```python
from build123d import *

# Parameters (mm, degrees)
SKETCH2_W           = 124
SKETCH2_H           = 45
BOSS_EXTRUDE3_DEPTH = 10
SKETCH4_W           = 100
SKETCH4_H           = 45
CUT_EXTRUDE1_DEPTH  = 7
CUT_EXTRUDE2_REACH  = 68.71
SKETCH5_R           = 1.55
SKETCH6_W           = 10.2
SKETCH6_H           = 41.4
CUT_EXTRUDE3_DEPTH  = 7.5
SKETCH7_R           = 1.5
BOSS_EXTRUDE4_DEPTH = 4


with BuildPart() as part:
    # Sketch2 → Boss-Extrude3 (new body)
    with BuildSketch(Plane(origin=(0, 0, 0), x_dir=(1, 0, 0), z_dir=(0, 1, 0))):
        Rectangle(SKETCH2_W, SKETCH2_H)
    extrude(amount=BOSS_EXTRUDE3_DEPTH)

    # Sketch4 → Cut-Extrude1 (cut)
    with BuildSketch(Plane(origin=(0, 10, 0), x_dir=(1, 0, 0), z_dir=(0, 1, 0))):
        Rectangle(SKETCH4_W, SKETCH4_H)
    extrude(amount=-CUT_EXTRUDE1_DEPTH, mode=Mode.SUBTRACT)

    # Sketch5 → Cut-Extrude2 (cut, up to next)
    with BuildSketch(Plane(origin=(0, 10, 0), x_dir=(1, 0, 0), z_dir=(0, 1, 0)), mode=Mode.PRIVATE) as cut_extrude2_sk1:
        with Locations(Location((-57, 12, 0), (0, 0, 270))):
            Circle(SKETCH5_R)
    cut_extrude2_tool1 = extrude(cut_extrude2_sk1.sketch, amount=-CUT_EXTRUDE2_REACH, mode=Mode.PRIVATE) & part.part
    # Sketch5 → Cut-Extrude2 (cut, up to next)
    with BuildSketch(Plane(origin=(0, 10, 0), x_dir=(1, 0, 0), z_dir=(0, 1, 0)), mode=Mode.PRIVATE) as cut_extrude2_sk2:
        with Locations(Location((-57, -12, 0), (0, 0, 270))):
            Circle(SKETCH5_R)
    cut_extrude2_tool2 = extrude(cut_extrude2_sk2.sketch, amount=-CUT_EXTRUDE2_REACH, mode=Mode.PRIVATE) & part.part
    # Sketch5 → Cut-Extrude2 (cut, up to next)
    with BuildSketch(Plane(origin=(0, 10, 0), x_dir=(1, 0, 0), z_dir=(0, 1, 0)), mode=Mode.PRIVATE) as cut_extrude2_sk3:
        with Locations(Location((57, -12, 0), (0, 0, 270))):
            Circle(SKETCH5_R)
    cut_extrude2_tool3 = extrude(cut_extrude2_sk3.sketch, amount=-CUT_EXTRUDE2_REACH, mode=Mode.PRIVATE) & part.part
    # Sketch5 → Cut-Extrude2 (cut, up to next)
    with BuildSketch(Plane(origin=(0, 10, 0), x_dir=(1, 0, 0), z_dir=(0, 1, 0)), mode=Mode.PRIVATE) as cut_extrude2_sk4:
        with Locations(Location((57, 12, 0), (0, 0, 270))):
            Circle(SKETCH5_R)
    cut_extrude2_tool4 = extrude(cut_extrude2_sk4.sketch, amount=-CUT_EXTRUDE2_REACH, mode=Mode.PRIVATE) & part.part
    add(cut_extrude2_tool1.solids().sort_by_distance((-57, 10, -12))[0], mode=Mode.SUBTRACT)
    add(cut_extrude2_tool2.solids().sort_by_distance((-57, 10, 12))[0], mode=Mode.SUBTRACT)
    add(cut_extrude2_tool3.solids().sort_by_distance((57, 10, 12))[0], mode=Mode.SUBTRACT)
    add(cut_extrude2_tool4.solids().sort_by_distance((57, 10, -12))[0], mode=Mode.SUBTRACT)

    # Sketch6 → Cut-Extrude3 (cut)
    with BuildSketch(Plane.XZ):
        with Locations((-56.9, 0)):
            Rectangle(SKETCH6_W, SKETCH6_H)
        with Locations((56.9, 0)):
            Rectangle(SKETCH6_W, SKETCH6_H)
    extrude(amount=-CUT_EXTRUDE3_DEPTH, mode=Mode.SUBTRACT)

    # Sketch7 → Boss-Extrude4 (add)
    # profile 1 of 4: a face of its own
    with BuildSketch(Plane(origin=(0, 3, 0), x_dir=(1, 0, 0), z_dir=(0, 1, 0))):
        with BuildLine():
            Line((-50, -17.5), (-44.5, -17.5))
            Line((-44.5, -17.5), (-44.5, -14.5))
            ThreePointArc((-44.5, -14.5), (-45.232233047, -12.732233047), (-47, -12))
            Line((-47, -12), (-50, -12))
            Line((-50, -12), (-50, -17.5))
        make_face()
        with Locations(Location((-47, -14.5, 0), (0, 0, 270))):
            Circle(SKETCH7_R, mode=Mode.SUBTRACT)
    # profile 2 of 4: a face of its own
    with BuildSketch(Plane(origin=(0, 3, 0), x_dir=(1, 0, 0), z_dir=(0, 1, 0))):
        with BuildLine():
            Line((44.5, -14.5), (44.5, -17.5))
            Line((44.5, -17.5), (50, -17.5))
            Line((50, -17.5), (50, -12))
            Line((50, -12), (47, -12))
            ThreePointArc((47, -12), (45.232233047, -12.732233047), (44.5, -14.5))
        make_face()
        with Locations(Location((47, -14.5, 0), (0, 0, 270))):
            Circle(SKETCH7_R, mode=Mode.SUBTRACT)
    # profile 3 of 4: a face of its own
    with BuildSketch(Plane(origin=(0, 3, 0), x_dir=(1, 0, 0), z_dir=(0, 1, 0))):
        with BuildLine():
            Line((-50, 17.5), (-50, 12))
            Line((-50, 12), (-47, 12))
            ThreePointArc((-47, 12), (-45.232233047, 12.732233047), (-44.5, 14.5))
            Line((-44.5, 14.5), (-44.5, 17.5))
            Line((-44.5, 17.5), (-50, 17.5))
        make_face()
        with Locations(Location((-47, 14.5, 0), (0, 0, 270))):
            Circle(SKETCH7_R, mode=Mode.SUBTRACT)
    # profile 4 of 4: a face of its own
    with BuildSketch(Plane(origin=(0, 3, 0), x_dir=(1, 0, 0), z_dir=(0, 1, 0))):
        with BuildLine():
            Line((47, 12), (50, 12))
            Line((50, 12), (50, 17.5))
            Line((50, 17.5), (44.5, 17.5))
            Line((44.5, 17.5), (44.5, 14.5))
            ThreePointArc((44.5, 14.5), (45.232233047, 12.732233047), (47, 12))
        make_face()
        with Locations(Location((47, 14.5, 0), (0, 0, 270))):
            Circle(SKETCH7_R, mode=Mode.SUBTRACT)
    extrude(amount=BOSS_EXTRUDE4_DEPTH)


solid = part.part
```
Check sheet for the modelled part. Datum: model origin and axes. Units: mm. A direction names the side the tool comes from. Coordinates: 2 decimals unless noted, no trailing zeros. Write each loop counter-clockwise with the first axis right and the second up, starting at its lowest first coordinate (ties: lowest second). Pieces come first, ordered by that corner, then holes. Notation, with made-up numbers: (48, -5) -> (98, -5) arc R14 cw to (98, 1) -> close; hole circle Ø11 at (66.5, 12.25). An arc over 180 degrees is marked (long way). Use a Markdown table: item, result.
1. Tool access check on faces 4 (the flat face through (44.5, 5, -16)), 5 (the cylindrical face through (-48.464, 4.972, -14.825)), 6 (the flat face through (-47, 5, 17.5)). Record the directions out of +Z, -Z, +X, -X, +Y, -Y that give a thin tool (end or side, any length) a straight path to the whole face; none if there is none.
Reported:
| item | result |
|---|---|
| face 4 | +Z, -Z, +Y |
| face 5 | +Y |
| face 6 | +Z, +Y |
2. Sectioned sample at D-D (x = 33.5). Enter the section's corners in (y, z), plus the area to 3 significant figures.
Reported:
| item | result |
|---|---|
| outline | (0, -22.5) -> (3, -22.5) -> (3, 22.5) -> (0, 22.5) -> close |
| area | 135 mm2 |
3. Sectioned sample at C-C (z = 1.5). Enter the section's corners in (x, y), plus the area to 3 significant figures.
Reported:
| item | result |
|---|---|
| outline | (-62, 7.5) -> (-51.8, 7.5) -> (-51.8, 0) -> (51.8, 0) -> (51.8, 7.5) -> (62, 7.5) -> (62, 10) -> (50, 10) -> (50, 3) -> (-50, 3) -> (-50, 10) -> (-62, 10) -> close |
| area | 387 mm2 |
4. Go/stop test with flat-tipped pins: pin 1 Ø5 at (x, z) = (47, -14.5) entering from +Y; pin 2 Ø3.5 at (y, z) = (5.5, -16.5) entering from -X; pin 3 Ø1.5 at (x, y) = (49, 5.5) entering from -Z; pin 4 Ø6 at (x, y) = (-31.5, 7) entering from -Z. Record where each tip stops, or that it passes through.
Reported:
| item | result |
|---|---|
| pin 1 | stops at y = 7 |
| pin 2 | stops at x = -51.8 |
| pin 3 | stops at z = -17.5 |
| pin 4 | passes through |
5. Sectioned sample at B-B (x = 57). Enter the section's corners in (y, z), plus the area to 3 significant figures.
Reported:
| item | result |
|---|---|
| outline | (0, -22.5) -> (10, -22.5) -> (10, -13.55) -> (7.5, -13.55) -> (7.5, -20.7) -> (0, -20.7) -> close; (0, 20.7) -> (7.5, 20.7) -> (7.5, 13.55) -> (10, 13.55) -> (10, 22.5) -> (0, 22.5) -> close; (7.5, -10.45) -> (10, -10.45) -> (10, 10.45) -> (7.5, 10.45) -> close |
| area | 124 mm2 |
6. Scan lines: line 1 along X through (y, z) = (8.85, -12); line 2 along X through (y, z) = (5.8, -14.5); line 3 along X through (y, z) = (6, -9.5). Record each from-to range of solid material in increasing order.
Reported:
| item | result |
|---|---|
| line 1 | x = -62 to -58.55, -55.45 to -50, 50 to 55.45, 58.55 to 62 |
| line 2 | x = -51.8 to -48.5, -45.5 to -44.5, 44.5 to 45.5, 48.5 to 51.8 |
| line 3 | x = -51.8 to -50, 50 to 51.8 |
7. Sectioned sample at A-A (y = 8.75). Enter the section's corners in (x, z).
Reported:
| item | result |
|---|---|
| outline | (-62, -22.5) -> (-50, -22.5) -> (-50, 22.5) -> (-62, 22.5) -> close; (50, -22.5) -> (62, -22.5) -> (62, 22.5) -> (50, 22.5) -> close; hole circle Ø3.1 at (-57, -12); hole circle Ø3.1 at (-57, 12); hole circle Ø3.1 at (57, -12); hole circle Ø3.1 at (57, 12) |
8. Release check for a two-part mould opening along X. For faces 1 (the flat face through (-56, 10, 0)), 2 (the flat face through (-1, 3, 0)), 3 (the flat face through (47, 5, 17.5)) record: pulls with the +X half, pulls with the -X half, needs draft (parallel to the pull), parting line crosses it, or undercut.
Reported:
| item | result |
|---|---|
| face 1 | needs draft |
| face 2 | undercut |
| face 3 | undercut |
